For this review, take the finished solid that the model builds, in its own axes (mm). A direction names the side the tool comes from. Coordinates: 2 decimals unless noted, no trailing zeros. Write each loop counter-clockwise with the first axis right and the second up, starting at its lowest first coordinate (ties: lowest second). Pieces come first, ordered by that corner, then holes. Notation, with made-up numbers: (32, 48) - (68, 48) arc R23 ccw to (68, 66) - close; hole circle Ø10 at (0.5, 46.25). An arc over 180 degrees is marked (long way). Write each question's results on one line, items separated by ' | '.
from build123d import *

# Parameters (mm, degrees)
SKETCH1_R           = 55
SKETCH1_R_2         = 14.5
BOSS_EXTRUDE1_DEPTH = 20
SKETCH2_R           = 20.75
CUT_EXTRUDE1_DEPTH  = 10
SKETCH4_R           = 2
CUT_EXTRUDE2_DEPTH  = 20
SKETCH6_R           = 5
CUT_EXTRUDE3_DEPTH  = 5


with BuildPart() as part:
    # Sketch1 → Boss-Extrude1 (new body)
    with BuildSketch(Plane(origin=(0, 0, 0), x_dir=(1, 0, 0), z_dir=(0, 1, 0))):
        Circle(SKETCH1_R)
        Circle(SKETCH1_R_2, mode=Mode.SUBTRACT)
    extrude(amount=BOSS_EXTRUDE1_DEPTH)

    # Sketch2 → Cut-Extrude1 (cut)
    with BuildSketch(Plane(origin=(0, 20, 0), x_dir=(1, 0, 0), z_dir=(0, 1, 0))):
        Circle(SKETCH2_R)
    extrude(amount=-CUT_EXTRUDE1_DEPTH, mode=Mode.SUBTRACT)

    # Sketch4 → Cut-Extrude2 (cut)
    with BuildSketch(Plane(origin=(0, 20, 0), x_dir=(1, 0, 0), z_dir=(0, 1, 0))):
        with Locations((0, 45)):
            Circle(SKETCH4_R)
        with Locations((45, 0)):
            Circle(SKETCH4_R)
        with Locations((0, -45)):
            Circle(SKETCH4_R)
        with Locations((-45, 0)):
            Circle(SKETCH4_R)
    extrude(amount=-CUT_EXTRUDE2_DEPTH, mode=Mode.SUBTRACT)

    # Sketch6 → Cut-Extrude3 (cut)
    with BuildSketch(Plane.XZ):
        with Locations((0, 45)):
            Circle(SKETCH6_R)
        with Locations((45, 0)):
            Circle(SKETCH6_R)
        with Locations((0, -45)):
            Circle(SKETCH6_R)
        with Locations((-45, 0)):
            Circle(SKETCH6_R)
    extrude(amount=-CUT_EXTRUDE3_DEPTH, mode=Mode.SUBTRACT)


solid = part.part
Q1. Take a section at B-B on x = 0. State the section outline as (y, z) points.
Results found:
outline: (0, -55) - (20, -55) - (20, -47) - (5, -47) - (5, -50) - (0, -50) - close; (0, -40) - (5, -40) - (5, -43) - (20, -43) - (20, -20.75) - (10, -20.75) - (10, -14.5) - (0, -14.5) - close; (0, 14.5) - (10, 14.5) - (10, 20.75) - (20, 20.75) - (20, 43) - (5, 43) - (5, 40) - (0, 40) - close; (0, 50) - (5, 50) - (5, 47) - (20, 47) - (20, 55) - (0, 55) - close
Q2. For pin 1 (4 mm diameter, centred on x = -6, y = 12.5, fed in from -Z); pin 2 (12 mm diameter, centred on y = 3.5, z = 21.5, fed in from -X); pin 3 (12 mm diameter, centred on x = 5.5, y = 12.5, fed in from -Z); pin 4 (8 mm diameter, centred on x = -47, z = 1.5, fed in from -Y), all flat-tipped, find the tip position at first contact; note any pin that passes through.
Results found:
pin 1: z = -54.85 | pin 2: x = -52.77 | pin 3: z = -55 | pin 4: y = 0
Q3. Take a section at C-C on z = 0. State the section outline as (x, y) points, plus the area to 4 significant figures.
Results found:
outline: (-55, 0) - (-50, 0) - (-50, 5) - (-47, 5) - (-47, 20) - (-55, 20) - close; (-43, 5) - (-40, 5) - (-40, 0) - (-14.5, 0) - (-14.5, 10) - (-20.75, 10) - (-20.75, 20) - (-43, 20) - close; (14.5, 0) - (40, 0) - (40, 5) - (43, 5) - (43, 20) - (20.75, 20) - (20.75, 10) - (14.5, 10) - close; (47, 5) - (50, 5) - (50, 0) - (55, 0) - (55, 20) - (47, 20) - close | area: 1,275 mm2
Q4. For faces 4 (the face through (43, 13, 0)), 5 (the face through (40, 2, 0)), 6 (the face through (19.8, 15.1, -6.2)), list the 3-axis set-ups (+Z, -Z, +X, -X, +Y, -Y) from which the entire face can be reached by the end or side of a thin tool; tool diameter is ignored.
Results found:
face 4: +Y, -Y | face 5: -Y | face 6: +Y
Q5. Mouldability with a two-part tool opening along X and no side actions: class faces 1 (the face through (-11.923, 9.86, 53.692)), 2 (the face through (-0.651, 2.465, -40.043)), 3 (the face through (11, 0, 11)) as pulls with the +X half, pulls with the -X half, needs draft (parallel to the pull), parting line crosses it, or undercut.
Results found:
face 1: parting line crosses it | face 2: undercut | face 3: needs draft
Q6. Take a section at D-D on x = -45. State the section outline as (y, z) points, plus the area to 3 significant figures.
Results found:
outline: (0, -31.62) - (20, -31.62) - (20, -2) - (5, -2) - (5, -5) - (0, -5) - close; (0, 5) - (5, 5) - (5, 2) - (20, 2) - (20, 31.62) - (0, 31.62) - close | area: 1,150 mm2
Q7. Wall thickness on line 1 along X through (y, z) = (10.75, 0); line 2 along Z through (x, y) = (0, 9); line 3 along Z through (x, y) = (0, 2.85): over which ranges is each line inside the solid? List them lowest first. Write a range as from..to.
Results found:
line 1: -55..-47, -43..-20.75, 20.75..43, 47..55 | line 2: -55..-47, -43..-14.5, 14.5..43, 47..55 | line 3: -55..-50, -40..-14.5, 14.5..40, 50..55
Q8. Take a section at A-A on y = 7. State the section outline as (x, z) points.
Results found:
outline: circle Ø110 at (0, 0); hole circle Ø4 at (-45, 0); hole circle Ø29 at (0, 0); hole circle Ø4 at (0, -45); hole circle Ø4 at (0, 45); hole circle Ø4 at (45, 0)
